For this review, take the finished solid that the model builds, in its own axes (mm). Face numbers are marked on the shaded views. A direction names the side the tool comes from. Coordinates: 2 decimals unless noted, no trailing zeros. Loops run counter-clockwise (first coordinate to the right, second up) from the corner with the lowest first, then second, coordinate; pieces in that order, holes last.
```python
from build123d import *

# Parameters (mm, degrees)
F1_DEPTH      = 21.59
F2_R          = 4.7625
F3_DEPTH      = 76.201
F4_R          = 12.7
F5_DEPTH      = 9.779
F5_DEPTH_BACK = 25.147


with BuildPart() as f1:
    # F0 (on Front) → F1 (new body, symmetric)
    with BuildSketch(Plane.XZ):
        Polygon((-40.64, 0), (0, 0), (0, 34.925), (-28.3972, 34.925), (-28.3972, 64.77), (-60.325, 64.77), (-60.325, 124.206), (-76.2, 124.206), (-76.2, 25.146), (-40.64, 25.146), align=None)
    extrude(amount=F1_DEPTH, both=True)

    # F2 (on face) → F3 (cut, through all)
    with BuildSketch(Plane(origin=(-76.2, 0, 0), x_dir=(0, -1, 0), z_dir=(-1, 0, 0))):
        with Locations((0, 114.681)):
            Circle(F2_R)
        with Locations((0, 79.756)):
            Circle(F2_R)
    extrude(amount=-F3_DEPTH, mode=Mode.SUBTRACT)

    # F4 (on face) → F5 (cut, two sides)
    with BuildSketch(Plane(origin=(0, 0, 25.146), x_dir=(1, 0, 0), z_dir=(0, 0, -1))) as f5_sk:
        with Locations((-58.42, 0)):
            Circle(F4_R)
        with Locations((-20.32, 0)):
            Circle(F4_R)
    extrude(amount=-F5_DEPTH, mode=Mode.SUBTRACT)
    extrude(f5_sk.sketch, amount=F5_DEPTH_BACK, mode=Mode.SUBTRACT)


solid = f1.part
```
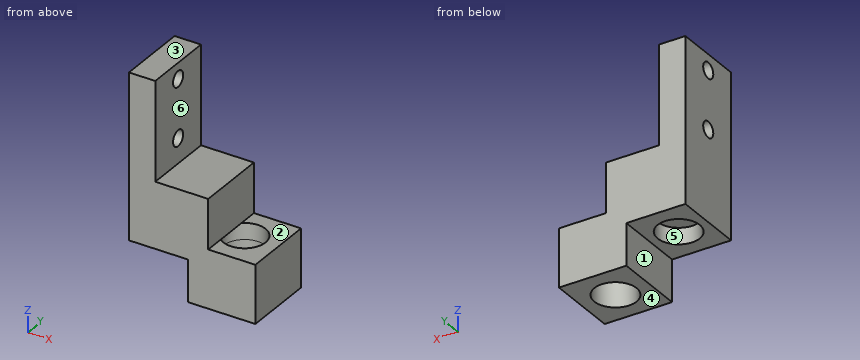
Q1. The part is to be moulded in two halves that separate along X. For the marked faces 4, 5 and 6, say which applies: +X half, -X half, draft (parallel to the pull), parting line (faces both ways), or undercut.
Q2. Consider section B-B (x = -20.32). State the section outline as (y, z) points (3 decimals), then the cut area to 3 significant figures.
Q3. Consider section A-A (y = 0). State the section outline as (x, z) points (1 decimal), then the cut area to 3 significant figures.
Q4. Consider section C-C (z = 76.5). State the section outline as (x, y) points (3 decimals).
Q5. Consider section D-D (y = -19). State the section outline as (x, z) points (3 decimals).
Q6. Wall thickness on probe 1 along Z at (x, y) = (-66, 0) (1 decimal); probe 2 along X at (y, z) = (0, 30); probe 3 along Y at (x, z) = (-20.32, 31.25): over which ranges is each line inside the solid? List them lowest first.
Q7. For pin 1 Ø15 at (y, z) = (0, 114.681) entering from +X (3 decimals); pin 2 Ø8 at (y, z) = (0.5, 62) entering from +X; pin 3 Ø10.5 at (x, y) = (-61.5, -10.5) entering from -Z, all flat-tipped, find the tip position at first contact; note any pin that passes through.
Q8. Machinability: for the marked faces 1, 2 and 3, which of the approach directions +Z, -Z, +X, -X, +Y, -Y give a long, thin tool a straight path to every point of the face, cutting with its end or side? Answer none if there is none.
Model answer:
1. face 4: draft
1. face 5: undercut
1. face 6: +X half
2. outline: (-21.59, 0) - (-12.7, 0) - (-12.7, 34.925) - (-21.59, 34.925) - close; (12.7, 0) - (21.59, 0) - (21.59, 34.925) - (12.7, 34.925) - close
2. area: 621 mm2
3. outline: (-76.2, 25.1) - (-71.1, 25.1) - (-71.1, 34.9) - (-45.7, 34.9) - (-45.7, 25.1) - (-40.6, 25.1) - (-40.6, 0) - (-33, 0) - (-33, 34.9) - (-28.4, 34.9) - (-28.4, 64.8) - (-60.3, 64.8) - (-60.3, 75) - (-76.2, 75) - close; (-76.2, 84.5) - (-60.3, 84.5) - (-60.3, 109.9) - (-76.2, 109.9) - close; (-76.2, 119.4) - (-60.3, 119.4) - (-60.3, 124.2) - (-76.2, 124.2) - close; (-7.6, 0) - (0, 0) - (0, 34.9) - (-7.6, 34.9) - close
3. area: 2,700 mm2
4. outline: (-76.2, -21.59) - (-60.325, -21.59) - (-60.325, -3.476) - (-76.2, -3.476) - close; (-76.2, 3.476) - (-60.325, 3.476) - (-60.325, 21.59) - (-76.2, 21.59) - close
5. outline: (-76.2, 25.146) - (-40.64, 25.146) - (-40.64, 0) - (0, 0) - (0, 34.925) - (-28.397, 34.925) - (-28.397, 64.77) - (-60.325, 64.77) - (-60.325, 124.206) - (-76.2, 124.206) - close
6. probe 1: z = 34.9 to 75, 84.5 to 109.9, 119.4 to 124.2
6. probe 2: x = -76.2 to -71.12, -45.72 to -33.02, -7.62 to 0
6. probe 3: y = -21.59 to -12.7, 12.7 to 21.59
7. pin 1: stops at x = -60.325
7. pin 2: stops at x = -28.4
7. pin 3: stops at z = 25.15
8. face 1: -Z, -X, +Y, -Y
8. face 2: +Z, +X, +Y, -Y
8. face 3: +Z, +X, -X, +Y, -Y
